from build123d import *

# Parameters (mm, degrees)
ESQUISSE1_R        = 1.25
ESQUISSE1_R_2      = 1.5
BOSS_EXTRU_1_DEPTH = 25
ESQUISSE3_R        = 1.5
BOSS_EXTRU_2_DEPTH = 2.5


with BuildPart() as part:
    # Esquisse1 → Boss.-Extru.1 (new, symmetric)
    with BuildSketch(Plane.XY):
        with BuildLine():
            Line((0, 4), (30.413812651, 4))
            ThreePointArc((30.413812651, 4), (34.413812651, 0), (30.413812651, -4))
            Line((30.413812651, -4), (0, -4))
            ThreePointArc((0, -4), (-4, 0), (0, 4))
        make_face()
        Circle(ESQUISSE1_R, mode=Mode.SUBTRACT)
        with Locations((30.413812651, 0)):
            Circle(ESQUISSE1_R_2, mode=Mode.SUBTRACT)
    extrude(amount=BOSS_EXTRU_1_DEPTH, both=True)

    # Esquisse3 → Boss.-Extru.2 (add, symmetric)
    with BuildSketch(Plane.XY):
        with BuildLine():
            Line((33.877914267, -2), (28.877914267, -10.660254038))
            ThreePointArc((28.877914267, -10.660254038), (25.149451096, -12.651508599), (21.716189443, -10.185895741))
            ThreePointArc((21.716189443, -10.185895741), (18.033559179, -5.689132338), (12.472131421, -4))
            Line((12.472131421, -4), (30.413812651, -4))
            ThreePointArc((30.413812651, -4), (32.413812651, -3.464101615), (33.877914267, -2))
        make_face()
        with Locations((25.413812651, -8.660254038)):
            Circle(ESQUISSE3_R, mode=Mode.SUBTRACT)
    extrude(amount=BOSS_EXTRU_2_DEPTH, both=True)

    # Esquisse4 → Enl_vement de mati_re-R_volution1 (revolve, cut)
    with BuildSketch(Plane(origin=(0, 0, 0), x_dir=(1, 0, 0), z_dir=(0, 1, 0)), mode=Mode.PRIVATE) as enl_vement_de_mati_re_r_volution1_sk:
        with BuildLine():
            Line((0, 21), (5, 21))
            ThreePointArc((5, 21), (8.043807145, 19.966766701), (9.829629131, 17.294095226))
            Line((9.829629131, 17.294095226), (14.11681621, 1.294095226))
            ThreePointArc((14.11681621, 1.294095226), (14.287187079, 0), (14.11681621, -1.294095226))
            Line((14.11681621, -1.294095226), (9.829629131, -17.294095226))
            ThreePointArc((9.829629131, -17.294095226), (8.043807145, -19.966766701), (5, -21))
            Line((5, -21), (0, -21))
            Line((0, -21), (0, 21))
        make_face()
        with BuildLine():
            Line((34.413812651, 25), (6.221001618, 25))
            ThreePointArc((6.221001618, 25), (7.680759567, 24.782165485), (9.01332325, 24.147642692))
            Line((9.01332325, 24.147642692), (17.621491019, 18.352357308))
            ThreePointArc((17.621491019, 18.352357308), (18.954054703, 17.717834515), (20.413812651, 17.5))
            Line((20.413812651, 17.5), (34.413812651, 17.5))
            Line((34.413812651, 17.5), (34.413812651, 25))
        make_face()
        with BuildLine():
            Line((17.621491019, -18.352357308), (9.01332325, -24.147642692))
            ThreePointArc((9.01332325, -24.147642692), (7.680759567, -24.782165485), (6.221001618, -25))
            Line((6.221001618, -25), (34.413812651, -25))
            Line((34.413812651, -25), (34.413812651, -17.5))
            Line((34.413812651, -17.5), (20.413812651, -17.5))
            ThreePointArc((20.413812651, -17.5), (18.954054703, -17.717834515), (17.621491019, -18.352357308))
        make_face()
    revolve(enl_vement_de_mati_re_r_volution1_sk.sketch.rotate(Axis((0, 0, -21), (0, 0, 1)), 180), axis=Axis((0, 0, -21), (0, 0, 1)), mode=Mode.SUBTRACT)


solid = part.part
Can you work these out from the model? Positions are in its coordinate system, mm. A direction names the side the tool comes from. Coordinates: 2 decimals unless noted, no trailing zeros. Write each loop counter-clockwise with the first axis right and the second up, starting at its lowest first coordinate (ties: lowest second). Pieces come first, ordered by that corner, then holes. Notation, with made-up numbers: (5, 77) -> (48, 77) arc R19 cw to (48, 84) -> close; hole circle Ø7 at (45.25, 59). An arc over 180 degrees is marked (long way). Write each question's results on one line, items separated by ' | '. Start each with the question number.
Q1. We'd pull the mould along Z, two halves only. Please class faces 1 (the face through (27, 0, -17.5)), 2 (the face through (2, 0, 21)), 3 (the face through (31.845, 0.451, -0.245)): +Z half, -Z half, draft (parallel to the pull), parting line (faces both ways), or undercut.
Q2. If I drill on probe 1 along Y at (x, z) = (0, -22); probe 2 along Z at (x, y) = (4, 1); probe 3 along Z at (x, y) = (23, -8), over which ranges is the centre line in solid material (lowest first)?
Q3. Imagine slicing it at D-D (y = 0). State how many separate pieces and enclosed holes the cut face has, then the cut area to 3 significant figures.
Q4. On a 3-axis mill with a long thin cutter (end or side, diameter ignored), from which of +Z, -Z, +X, -X, +Y, -Y can I reach the whole of each face in a straight line? I mean faces 4 (the face through (19, -4, 14)), 5 (the face through (34.413, 0.088, 0.245)), 6 (the face through (27, 0, 17.5)), 7 (the face through (12, -0.1, -9.2)), 8 (the face through (1, 1, -25)). Say none if no direction works.
Q5. Imagine slicing it at B-B (z = 0). Write out the boundary of the cut face in (x, y).
Q6. I'm going to push flat-ended pins straight in: pin 1 (1.5 mm diameter, centred on x = 0, y = 0, fed in from +Z); pin 2 (2 mm diameter, centred on x = 25.5, y = -8, fed in from +Z); pin 3 (8.5 mm diameter, centred on x = 27.5, y = -6, fed in from -Z); pin 4 (18 mm diameter, centred on x = 19.5, z = 18.5, fed in from -Y). Where does each tip first touch, or does it pass through?
Q7. Imagine slicing it at A-A (x = 24.5). Write out the boundary of the cut face in (y, z).
Q8. Imagine slicing it at C-C (z = 6.5). Write out the boundary of the cut face in (x, y).
Taken from the geometry:
1) face 1: -Z half | face 2: undercut | face 3: draft
2) probe 1: y = -4 to -1.25, 1.25 to 4 | probe 2: z = -25 to -21, 21 to 25 | probe 3: z = -2.5 to 2.5
3) separate pieces: 4 | enclosed holes: 0 | area: 828 mm^2
4) face 4: +Z, +X, -X, -Y | face 5: +X | face 6: +Z, +X, +Y, -Y | face 7: -X | face 8: -Z, +X, -X, +Y, -Y
5) outline: (13.69, -4.07) arc R10 cw to (21.72, -10.19) arc R4 ccw to (28.88, -10.66) -> (33.88, -2) arc R4 ccw to (30.41, 4) -> (13.72, 4) arc R14.29 cw to start; hole circle Ø3 at (25.41, -8.66); hole circle Ø3 at (30.41, 0)
6) pin 1: passes through | pin 2: stops at z = 2.5 | pin 3: stops at z = -17.5 | pin 4: stops at y = -4
7) outline: (-12.55, -2.5) -> (-9.85, -2.5) -> (-9.85, 2.5) -> (-12.55, 2.5) -> close; (-7.47, -2.5) -> (-4, -2.5) -> (-4, -17.5) -> (4, -17.5) -> (4, 17.5) -> (-4, 17.5) -> (-4, 2.5) -> (-7.47, 2.5) -> close
8) outline: (12.08, -4) -> (30.41, -4) arc R4 ccw to (30.41, 4) -> (12.08, 4) arc R12.72 cw to start; hole circle Ø3 at (30.41, 0)
